Solid Edge part; units mm, degrees
sketch "Sketch1" plane through (0, 0, 0) normal (-1, 0, 0) x (0, -1, 0)
  line L0 (-75, -85) -> (75, -85)
  line L1 (75, -85) -> (75, 85)
  line L2 (75, 85) -> (-75, 85)
  line L3 (-75, 85) -> (-75, -85)
extrude "Protrusion1" add sketch "Sketch1" against normal blind 86
sketch "Sketch2" plane through (43, 0, 85) normal (0, 0, 1) x (0, 1, 0)
  circle A0 centre (-70.1242, -27.7474) radius 1.5
  circle A1 centre (69.4258, 37.5213) radius 1.5
  circle A2 centre (43.1098, -38.1411) radius 1.5
  line L0 (60.2973, 2.6541) -> (60.2973, -6.0172)
  arc A3 (57.2973, -9.0172) -> (60.2973, -6.0172) centre (57.2973, -6.0172) ccw
  line L1 (57.2973, -9.0172) -> (35.8941, -9.0172)
  arc A4 (32.8941, -6.0172) -> (35.8941, -9.0172) centre (35.8941, -6.0172) ccw
  line L2 (32.8941, -6.0172) -> (32.8941, 2.6541)
  line L3 (38.2443, 7.8768) -> (32.8941, 2.6541)
  line L4 (38.2443, 7.8768) -> (54.8198, 7.8768)
  line L5 (54.8198, 7.8768) -> (60.2973, 2.6541)
  circle A5 centre (-70.1242, 37.5213) radius 1.5
  line L6 (62.4771, -11.8883) -> (30.8651, -11.8883)
  arc A6 (30.8651, -11.8883) -> (29.8651, -10.8883) centre (30.8651, -10.8883) cw
  line L7 (29.8651, -10.8883) -> (29.8651, 10.7833)
  arc A7 (29.8651, 10.7833) -> (30.8651, 11.7833) centre (30.8651, 10.7833) cw
  line L8 (30.8651, 11.7833) -> (62.4771, 11.7833)
  arc A8 (63.4771, 10.7833) -> (62.4771, 11.7833) centre (62.4771, 10.7833) ccw
  line L9 (63.4771, 10.7833) -> (63.4771, -10.8883)
  arc A9 (63.4771, -10.8883) -> (62.4771, -11.8883) centre (62.4771, -10.8883) cw
  line L10 (27.5172, 10.4355) -> (14.6909, 10.4355)
  arc A10 (14.6909, 10.4355) -> (13.6909, 9.4355) centre (14.6909, 9.4355) ccw
  line L11 (13.6909, 9.4355) -> (13.6909, -9.035)
  arc A11 (13.6909, -9.035) -> (14.6909, -10.035) centre (14.6909, -9.035) ccw
  line L12 (14.6909, -10.035) -> (27.5172, -10.035)
  arc A12 (27.5172, -10.035) -> (28.5172, -9.035) centre (27.5172, -9.035) ccw
  line L13 (28.5172, -9.035) -> (28.5172, 9.4355)
  arc A13 (28.5172, 9.4355) -> (27.5172, 10.4355) centre (27.5172, 9.4355) ccw
  line L14 (26.0742, 7.7398) -> (16.3023, 7.7398)
  line L15 (16.3023, 7.7398) -> (16.3023, -7.1708)
  line L16 (16.3023, -7.1708) -> (26.0742, -7.1708)
  line L17 (26.0742, -7.1708) -> (26.0742, 7.7398)
  line L18 (70.3256, -36.7522) -> (68.4203, -36.7522)
  line L19 (68.4203, -36.7522) -> (67.4677, -38.4022)
  line L20 (67.4677, -38.4022) -> (68.4203, -40.0522)
  line L21 (68.4203, -40.0522) -> (70.3256, -40.0522)
  line L22 (70.3256, -40.0522) -> (71.2782, -38.4022)
  line L23 (71.2782, -38.4022) -> (70.3256, -36.7522)
  line L24 (62.9348, -36.7522) -> (61.0296, -36.7522)
  line L25 (61.0296, -36.7522) -> (60.077, -38.4022)
  line L26 (60.077, -38.4022) -> (61.0296, -40.0522)
  line L27 (61.0296, -40.0522) -> (62.9348, -40.0522)
  line L28 (62.9348, -40.0522) -> (63.8875, -38.4022)
  line L29 (63.8875, -38.4022) -> (62.9348, -36.7522)
  line L30 (55.7847, -36.7522) -> (53.8795, -36.7522)
  line L31 (53.8795, -36.7522) -> (52.9268, -38.4022)
  line L32 (52.9268, -38.4022) -> (53.8795, -40.0522)
  line L33 (53.8795, -40.0522) -> (55.7847, -40.0522)
  line L34 (55.7847, -40.0522) -> (56.7374, -38.4022)
  line L35 (56.7374, -38.4022) -> (55.7847, -36.7522)
  line L36 (55.7847, -32.7647) -> (53.8795, -32.7647)
  line L37 (53.8795, -32.7647) -> (52.9268, -34.4147)
  line L38 (52.9268, -34.4147) -> (53.8795, -36.0647)
  line L39 (53.8795, -36.0647) -> (55.7847, -36.0647)
  line L40 (55.7847, -36.0647) -> (56.7374, -34.4147)
  line L41 (56.7374, -34.4147) -> (55.7847, -32.7647)
  line L42 (62.9348, -32.7647) -> (61.0296, -32.7647)
  line L43 (61.0296, -32.7647) -> (60.077, -34.4147)
  line L44 (60.077, -34.4147) -> (61.0296, -36.0647)
  line L45 (61.0296, -36.0647) -> (62.9348, -36.0647)
  line L46 (62.9348, -36.0647) -> (63.8875, -34.4147)
  line L47 (63.8875, -34.4147) -> (62.9348, -32.7647)
  line L48 (70.3256, -32.7647) -> (68.4203, -32.7647)
  line L49 (68.4203, -32.7647) -> (67.4677, -34.4147)
  line L50 (67.4677, -34.4147) -> (68.4203, -36.0647)
  line L51 (68.4203, -36.0647) -> (70.3256, -36.0647)
  line L52 (70.3256, -36.0647) -> (71.2782, -34.4147)
  line L53 (71.2782, -34.4147) -> (70.3256, -32.7647)
extrude "Cutout1" cut sketch "Sketch2" against normal blind 30
sketch "Sketch3" plane through (43.0525, 46.6711, 55) normal (0, 0, 1) x (0, 1, 0)
  line L0 (-16.806, 10.8358) -> (-16.806, -10.8358)
  arc A0 (-16.806, -10.8358) -> (-15.806, -11.8358) centre (-15.806, -10.8358) ccw
  line L1 (-15.806, -11.8358) -> (15.806, -11.8358)
  arc A1 (16.806, -10.8358) -> (15.806, -11.8358) centre (15.806, -10.8358) cw
  line L2 (16.806, -10.8358) -> (16.806, 10.8358)
  arc A2 (16.806, 10.8358) -> (15.806, 11.8358) centre (15.806, 10.8358) ccw
  line L3 (15.806, 11.8358) -> (-15.806, 11.8358)
  arc A3 (-15.806, 11.8358) -> (-16.806, 10.8358) centre (-15.806, 10.8358) ccw
  line L4 (-31.9802, 10.488) -> (-19.1539, 10.488)
  arc A4 (-18.1539, 9.488) -> (-19.1539, 10.488) centre (-19.1539, 9.488) ccw
  line L5 (-18.1539, 9.488) -> (-18.1539, -8.9825)
  arc A5 (-19.1539, -9.9825) -> (-18.1539, -8.9825) centre (-19.1539, -8.9825) ccw
  line L6 (-19.1539, -9.9825) -> (-31.9802, -9.9825)
  arc A6 (-31.9802, -9.9825) -> (-32.9802, -8.9825) centre (-31.9802, -8.9825) cw
  line L7 (-32.9802, -8.9825) -> (-32.9802, 9.488)
  arc A7 (-31.9802, 10.488) -> (-32.9802, 9.488) centre (-31.9802, 9.488) ccw
extrude "ExtrudedProtrusion_22" add sketch "Sketch3" along normal blind 32
sketch "Sketch4" plane through (43.0525, 46.6711, 70) normal (0, 0, 1) x (0, -1, 0)
  line L0 (-13.6262, 5.9647) -> (-13.6262, -2.7066)
  line L1 (-13.6262, -2.7066) -> (-8.1487, -7.9293)
  line L2 (-8.1487, -7.9293) -> (8.4268, -7.9293)
  line L3 (8.4268, -7.9293) -> (13.777, -2.7066)
  line L4 (13.777, -2.7066) -> (13.777, 5.9647)
  arc A0 (10.777, 8.9647) -> (13.777, 5.9647) centre (10.777, 5.9647) cw
  line L5 (-10.6262, 8.9647) -> (10.777, 8.9647)
  arc A1 (-10.6262, 8.9647) -> (-13.6262, 5.9647) centre (-10.6262, 5.9647) ccw
  line L6 (20.5968, 7.1183) -> (30.3688, 7.1183)
  line L7 (30.3688, 7.1183) -> (30.3688, -7.7923)
  line L8 (30.3688, -7.7923) -> (20.5968, -7.7923)
  line L9 (20.5968, -7.7923) -> (20.5968, 7.1183)
extrude "ExtrudedCutout_39" cut sketch "Sketch4" along normal blind 45
sketch "Sketch5" plane through (42.7155, 21.1883, 70) normal (0, 0, 1) x (0, 1, 0)
  line L0 (-4.886, 7.4553) -> (4.886, 7.4553)
  line L1 (4.886, 7.4553) -> (4.886, -7.4553)
  line L2 (4.886, -7.4553) -> (-4.886, -7.4553)
  line L3 (-4.886, -7.4553) -> (-4.886, 7.4553)
extrude "Protrusion2" add sketch "Sketch5" along normal blind 30
sketch "Sketch6" plane through (42.7155, 16.3023, 93.5) normal (0, -1, 0) x (0, 0, 1)
  line L0 (-6.5, -7.4553) -> (-1.5337, -3.4507)
  arc A0 (-6.5, 7.4553) -> (-1.5337, -3.4507) centre (8.0884, 7.5147) ccw
  line L1 (-6.5, 7.4553) -> (6.5, 7.4553)
  line L2 (6.5, 7.4553) -> (6.5, -7.4553)
  line L3 (6.5, -7.4553) -> (-6.5, -7.4553)
extrude "ExtrudedCutout_40" cut sketch "Sketch6" against normal blind 15
Model file for the job. Use its own axes, mm. A direction names the side the tool comes from. Give positions to 0.01 mm unless a question says otherwise; leave off trailing zeros. Loops run counter-clockwise (first coordinate to the right, second up) from the corner with the lowest first, then second, coordinate; pieces in that order, holes last. Notation, with made-up numbers: (4.25, 18.25) -> (61.25, 18.25) arc R22 ccw to (61.25, 57.25) -> close; hole circle Ø4 at (32, 69.5). An arc over 180 degrees is marked (long way). Use a Markdown table: item, result. Add a question column.
(1) Slice it at B-B on x = 38. List the corners of the cut face in (y, z), and give its area (3 significant figures).
(2) Tool access for faces 5 (the flat face through (45, 60.297, 78)), 6 (the flat face through (46, 26.074, 88)), 7 (the flat face through (44, 16.302, 88)): list every direction of +Z, -Z, +X, -X, +Y, -Y with a clear straight run to the whole face (end or side of a thin tool).
(3) Drop flat-ended pins along their axis: pin 1 Ø1 at (x, y) = (82, 70) entering from +Z; pin 2 Ø2.5 at (x, y) = (81.5, 61) entering from +Z; pin 3 Ø12 at (x, y) = (38.5, 23) entering from +Z. Give the stop position or say it passes through.
(4) Slice it at D-D on x = 61.5. List the corners of the cut face in (y, z).
(5) Wall check: line 1 along Z through (x, y) = (75, -22); line 2 along Z through (x, y) = (47, 28). Give the ranges that are in metal, low to high.
(6) Slice it at C-C on y = -63.5. List the corners of the cut face in (x, z), and give its area (3 significant figures).
(7) Slice it at A-A on y = 48.5. List the corners of the cut face in (x, z), and give its area (3 significant figures).
(8) Mould opens along X. For faces 1 (the flat face through (35.123, 47, 78)), 2 (the flat face through (42, 75, 1)), 3 (the cylindrical face through (41.168, 21.12, 88.276)), 4 (the flat face through (37.698, 35.607, 78.381)) say: +X half, -X half, draft (parallel to the pull), parting line (faces both ways), or undercut.
Filled sheet:
| question | item | result |
|---|---|---|
| 1 | outline | (-75, -85) -> (75, -85) -> (75, 85) -> (63.48, 85) -> (63.48, 87) -> (57.84, 87) -> (57.84, 70) -> (35.3, 70) -> (35.3, 87) -> (29.87, 87) -> (29.87, 85) -> (28.52, 85) -> (28.52, 87) -> (26.07, 87) -> (26.07, 87.27) -> (16.3, 87.27) -> (16.3, 87) -> (13.69, 87) -> (13.69, 85) -> (-75, 85) -> close |
| 1 | area | 25,200 mm2 |
| 2 | face 5 | +Z |
| 2 | face 6 | +Z, +X, -X, +Y |
| 2 | face 7 | +Z, +X, -X, -Y |
| 3 | pin 1 | z = 55 |
| 3 | pin 2 | z = 85 |
| 3 | pin 3 | z = 90.35 |
| 4 | outline | (-75, -85) -> (75, -85) -> (75, 85) -> (-75, 85) -> close |
| 5 | line 1 | -85 to 85 |
| 5 | line 2 | -85 to 87 |
| 6 | outline | (0, -85) -> (86, -85) -> (86, 85) -> (0, 85) -> close |
| 6 | area | 14,600 mm2 |
| 7 | outline | (0, -85) -> (86, -85) -> (86, 85) -> (54.89, 85) -> (54.89, 87) -> (52.02, 87) -> (52.02, 70) -> (35.12, 70) -> (35.12, 87) -> (31.22, 87) -> (31.22, 85) -> (0, 85) -> close |
| 7 | area | 14,400 mm2 |
| 8 | face 1 | undercut |
| 8 | face 2 | draft |
| 8 | face 3 | -X half |
| 8 | face 4 | undercut |
